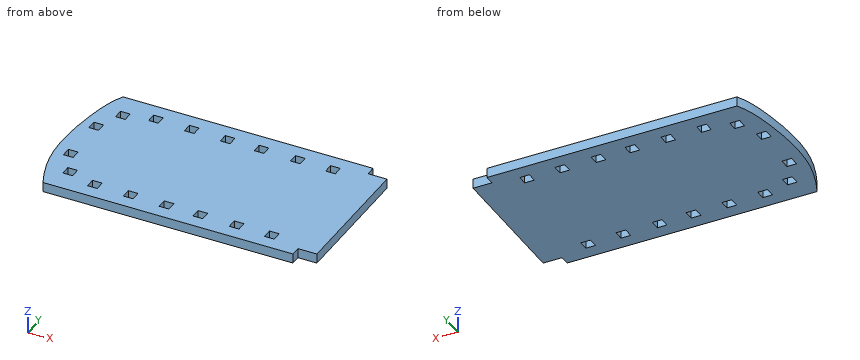
from build123d import *

# Parameters (mm, degrees)
BOSS_EXTRUDE1_DEPTH = 3.175
CUT_EXTRUDE1_DEPTH  = 3.175
SKETCH3_W           = 3.175
SKETCH3_H           = 3.175
CUT_EXTRUDE2_DEPTH  = 3.175
SKETCH4_W           = 9.525
SKETCH4_H           = 44.45
CUT_EXTRUDE3_DEPTH  = 3.175
CUT_EXTRUDE4_DEPTH  = 3.175


with BuildPart() as part:
    # Sketch1 → Boss-Extrude1 (new body)
    with BuildSketch(Plane.XY):
        with BuildLine():
            Line((47.738161277, 0), (129.678020066, 0))
            Line((129.678020066, 0), (129.678020066, -3.175))
            Line((129.678020066, -3.175), (145.421593995, -3.175))
            Line((145.421593995, -3.175), (145.421593995, -47.625))
            Line((145.421593995, -47.625), (129.678020066, -47.625))
            Line((129.678020066, -47.625), (129.678020066, -51.488987453))
            Line((129.678020066, -51.488987453), (47.738161277, -50.8))
            add(Edge.make_bspline(
                [(47.738161277, 0), (41.393133439, -1.711069928), (30.530442831, -9.367517151), (28.681444031, -25.622801065), (30.401296487, -42.131760993), (41.721917061, -48.493240739), (47.738161277, -50.8)],
                knots=[0, 0, 0, 0, 0.298782405, 0.512668788, 0.698134952, 1, 1, 1, 1], degree=3))
        make_face()
    extrude(amount=BOSS_EXTRUDE1_DEPTH)

    # Sketch2 → Cut-Extrude1 (cut)
    with BuildSketch(Plane.XY.offset(3.175)):
        with BuildLine():
            Line((47.738161277, 0), (25.94415126, 0))
            Line((25.94415126, 0), (25.94415126, -50.8))
            Line((25.94415126, -50.8), (47.738161277, -50.8))
            add(Edge.make_bspline(
                [(47.738161277, 0), (45.681525529, -3.647242432), (43.645083007, -12.887655636), (42.176101449, -25.699616702), (42.981732395, -39.048066027), (45.802728015, -46.725242417), (47.738161277, -50.8)],
                knots=[0, 0, 0, 0, 0.238683845, 0.536924902, 0.740325465, 1, 1, 1, 1], degree=3))
        make_face()
    extrude(amount=-CUT_EXTRUDE1_DEPTH, mode=Mode.SUBTRACT)

    # Sketch3 → Cut-Extrude2 (cut)
    with BuildSketch(Plane.XY.offset(3.175)):
        with Locations((61.621228186, -6.030517165)):
            Rectangle(SKETCH3_W, SKETCH3_H)
        with Locations((73.369830924, -6.030517165)):
            Rectangle(SKETCH3_W, SKETCH3_H)
        with Locations((85.118433661, -6.030517165)):
            Rectangle(SKETCH3_W, SKETCH3_H)
        with Locations((96.226203523, -6.030517165)):
            Rectangle(SKETCH3_W, SKETCH3_H)
        with Locations((108.110776123, -6.030517165)):
            Rectangle(SKETCH3_W, SKETCH3_H)
        with Locations((119.645767902, -6.030517165)):
            Rectangle(SKETCH3_W, SKETCH3_H)
        with Locations((52.144704899, -8.700654151)):
            Rectangle(SKETCH3_W, SKETCH3_H)
        with Locations((47.872485722, -17.351897985)):
            Rectangle(SKETCH3_W, SKETCH3_H)
        with Locations((47.872485722, -33.448102015)):
            Rectangle(SKETCH3_W, SKETCH3_H)
        with Locations((52.144704899, -42.099345849)):
            Rectangle(SKETCH3_W, SKETCH3_H)
        with Locations((61.621228186, -44.769482835)):
            Rectangle(SKETCH3_W, SKETCH3_H)
        with Locations((73.369830924, -44.769482835)):
            Rectangle(SKETCH3_W, SKETCH3_H)
        with Locations((85.118433661, -44.769482835)):
            Rectangle(SKETCH3_W, SKETCH3_H)
        with Locations((96.226203523, -44.769482835)):
            Rectangle(SKETCH3_W, SKETCH3_H)
        with Locations((108.110776123, -44.769482835)):
            Rectangle(SKETCH3_W, SKETCH3_H)
        with Locations((119.645767902, -44.769482835)):
            Rectangle(SKETCH3_W, SKETCH3_H)
    extrude(amount=-CUT_EXTRUDE2_DEPTH, mode=Mode.SUBTRACT)

    # Sketch4 → Cut-Extrude3 (cut)
    with BuildSketch(Plane.XY.offset(3.175)):
        with Locations((140.659093995, -25.4)):
            Rectangle(SKETCH4_W, SKETCH4_H)
    extrude(amount=-CUT_EXTRUDE3_DEPTH, mode=Mode.SUBTRACT)

    # Sketch5 → Cut-Extrude4 (cut)
    with BuildSketch(Plane.XY.offset(3.175)):
        Polygon((131.864975324, -55.496835694), (47.738161277, -50.8), (131.864975324, -50.8), align=None)
    extrude(amount=-CUT_EXTRUDE4_DEPTH, mode=Mode.SUBTRACT)


solid = part.part
The listing builds one solid part. Answer for the finished solid, in the listing's coordinates (mm). Coordinates: 2 decimals unless noted, no trailing zeros. Loops run counter-clockwise (first coordinate to the right, second up) from the corner with the lowest first, then second, coordinate; pieces in that order, holes last. Notation, with made-up numbers: (22.5, 30.5) -> (52.5, 30.5) arc R20 ccw to (52.5, 43.5) -> close; hole circle Ø4 at (63.5, -36). An arc over 180 degrees is marked (long way). Answer in a Markdown table with one row per item. Add a question column.
1. Consider line 1 (Y direction, x = 73, z = 2); line 2 (Y direction, x = 132, z = 1.1) (3 decimals); line 3 (X direction, y = -9, z = 1.3). Determine where each line is inside the solid, lowest interval first. Write a range as [from, to].
2. A flat-ended cylindrical pin translates along its axis: P1, Ø1, axis at y = -17, z = 1, coming from the -X side. Find the tip coordinate at first contact, or state that the pin passes through.
3. The part is cut by section A-A, the plane x = 73.5. Write down the section's boundary in (y, z) (3 decimals).
4. The part is cut by section B-B, the plane z = 2.3. Count the separate pieces of the cut face and the enclosed holes in it, then the cut area to 3 significant figures.
Answer below:
| question | item | result |
|---|---|---|
| 1 | line 1 | [-50.8, -46.36], [-43.18, -7.62], [-4.44, 0] |
| 1 | line 2 | [-47.625, -3.175] |
| 1 | line 3 | [44.61, 50.56], [53.73, 135.9] |
| 2 | P1 | x = 43.22 |
| 3 | outline | (-50.8, 0) -> (-46.357, 0) -> (-46.357, 3.175) -> (-50.8, 3.175) -> close; (-43.182, 0) -> (-7.618, 0) -> (-7.618, 3.175) -> (-43.182, 3.175) -> close; (-4.443, 0) -> (0, 0) -> (0, 3.175) -> (-4.443, 3.175) -> close |
| 4 | separate pieces | 1 |
| 4 | enclosed holes | 16 |
| 4 | area | 4,460 mm2 |
